```python
from build123d import *

# Parameters (mm, degrees)
SKETCH1_W                       = 152.4
SKETCH1_H                       = 101.6
BOSS_EXTRUDE1_DEPTH             = 46.99
SKETCH2_R                       = 17.145
CUT_EXTRUDE1_DEPTH              = 190.093574983
SKETCH2_2_R                     = 25.4
SKETCH2_2_R_2                   = 17.145
CUT_EXTRUDE3_DEPTH              = 12.446
TAP_DRILL_FOR_1_2_13_TAP1_D     = 10.71626
TAP_DRILL_FOR_1_2_13_TAP1_DEPTH = 19.05
TAP_DRILL_FOR_1_2_13_TAP1_TIP   = 3.219489309
TAP_DRILL_FOR_1_4_20_TAP1_D     = 5.1054
TAP_DRILL_FOR_1_4_20_TAP1_DEPTH = 13.706183098
TAP_DRILL_FOR_1_4_20_TAP1_TIP   = 1.533816902


with BuildPart() as part:
    # Sketch1 → Boss-Extrude1 (new body)
    with BuildSketch(Plane.XY):
        with Locations((76.2, 50.8)):
            Rectangle(SKETCH1_W, SKETCH1_H)
    extrude(amount=BOSS_EXTRUDE1_DEPTH)

    # Sketch2 → Cut-Extrude1 (cut, through all)
    with BuildSketch(Plane(origin=(0, 0, 0), x_dir=(-1, 0, 0), z_dir=(0, 0, -1))):
        with Locations((-76.2, 50.8)):
            Circle(SKETCH2_R)
    extrude(amount=-CUT_EXTRUDE1_DEPTH, mode=Mode.SUBTRACT)

    # Sketch2<2> → Cut-Extrude3 (cut)
    with BuildSketch(Plane(origin=(0, 0, 0), x_dir=(-1, 0, 0), z_dir=(0, 0, -1))):
        with Locations((-76.2, 50.8)):
            Circle(SKETCH2_2_R)
        with Locations((-76.2, 50.8)):
            Circle(SKETCH2_2_R_2, mode=Mode.SUBTRACT)
    cut_extrude3 = extrude(amount=-CUT_EXTRUDE3_DEPTH, mode=Mode.SUBTRACT)

    # Mirror2: Cut-Extrude3 across plane
    add(cut_extrude3.mirror(Plane(origin=(0, 0, 23.495), x_dir=(1, 0, 0), z_dir=(0, 0, -1))), mode=Mode.SUBTRACT)

    # Tap Drill for 1/2-13 Tap1
    with Locations(Plane(origin=(0, 0, 0), x_dir=(-1, 0, 0), z_dir=(0, -1, 0))):
        with Locations((-68.051669078, -23.495), (-29.951669078, -23.495)):
            Hole(TAP_DRILL_FOR_1_2_13_TAP1_D / 2, depth=TAP_DRILL_FOR_1_2_13_TAP1_DEPTH)
            with Locations((0, 0, -(TAP_DRILL_FOR_1_2_13_TAP1_DEPTH + TAP_DRILL_FOR_1_2_13_TAP1_TIP / 2))):  # 118° drill point
                Cone(0, TAP_DRILL_FOR_1_2_13_TAP1_D / 2, TAP_DRILL_FOR_1_2_13_TAP1_TIP, mode=Mode.SUBTRACT)

    # Tap Drill for 1/4-20 Tap1
    with Locations(Plane(origin=(50.8, 101.6, 0), x_dir=(0, 0, -1), z_dir=(0, 1, 0))):
        with Locations((-12.7, -47.625), (-12.7, -3.175)):
            Hole(TAP_DRILL_FOR_1_4_20_TAP1_D / 2, depth=TAP_DRILL_FOR_1_4_20_TAP1_DEPTH)
            with Locations((0, 0, -(TAP_DRILL_FOR_1_4_20_TAP1_DEPTH + TAP_DRILL_FOR_1_4_20_TAP1_TIP / 2))):  # 118° drill point
                Cone(0, TAP_DRILL_FOR_1_4_20_TAP1_D / 2, TAP_DRILL_FOR_1_4_20_TAP1_TIP, mode=Mode.SUBTRACT)


solid = part.part
```
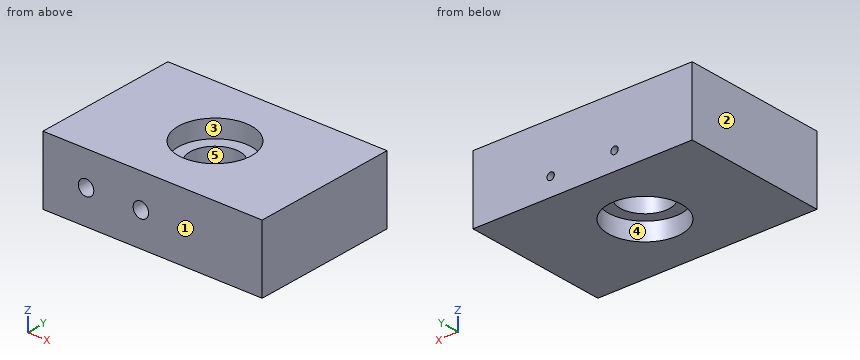
Source: CAD feature listing. Evaluate the final solid. Frame: model axes, mm. Face numbers are marked on the shaded views. A direction names the side the tool comes from. Give positions to 0.01 mm unless a question says otherwise; leave off trailing zeros. Loops run counter-clockwise (first coordinate to the right, second up) from the corner with the lowest first, then second, coordinate; pieces in that order, holes last. Notation, with made-up numbers: (2.25, -13.75) -> (13.25, -13.75) arc R26 cw to (13.25, 21.25) -> close; hole circle Ø3 at (32.5, -1.75). An arc over 180 degrees is marked (long way). Put each result on its own line as item: value. Start each with the question number.
1) Cut plane D-D (y = 6). Return loops of the section in (x, z) (3 decimals).
2) Cut plane A-A (x = 76.2). Return loops of the section in (y, z) (3 decimals).
3) Reachability of the marked faces 4 and 5 from +Z, -Z, +X, -X, +Y, -Y: full face, straight path, thin tool, end or side. Return the list, or none.
4) Cut plane B-B (y = 50.8). Return loops of the section in (x, z) (3 decimals).
5) Contact query for flat-ended pins moving along their axis: P1, Ø6.5, axis at x = 68.05, z = 23.5, coming from the -Y side; P2, Ø5, axis at x = 75, y = 67, coming from the -Z side; P3, Ø4.5, axis at x = 53.975, z = 12.7, coming from the +Y side. Output: stop coordinate, or through.
6) Cut plane C-C (y = 71). Return loops of the section in (x, z).
7) Material intervals for probe 1 along X at (y, z) = (98.75, 12.7); probe 2 along X at (y, z) = (6.5, 23); probe 3 along X at (y, z) = (50, 41), sorted ascending.
8) Draft query along X for the marked faces 1, 2 and 3. Return one class per face: released by +X, released by -X, zero draft, split by the parting line, or undercut.
Results are:
1. outline: (0, 0) -> (152.4, 0) -> (152.4, 46.99) -> (0, 46.99) -> close; hole circle Ø10.716 at (29.952, 23.495); hole circle Ø10.716 at (68.052, 23.495)
2. outline: (0, 0) -> (25.4, 0) -> (25.4, 12.446) -> (33.655, 12.446) -> (33.655, 34.544) -> (25.4, 34.544) -> (25.4, 46.99) -> (0, 46.99) -> close; (67.945, 12.446) -> (76.2, 12.446) -> (76.2, 0) -> (101.6, 0) -> (101.6, 46.99) -> (76.2, 46.99) -> (76.2, 34.544) -> (67.945, 34.544) -> close
3. face 4: -Z
3. face 5: +Z, -Z
4. outline: (0, 0) -> (50.8, 0) -> (50.8, 12.446) -> (59.055, 12.446) -> (59.055, 34.544) -> (50.8, 34.544) -> (50.8, 46.99) -> (0, 46.99) -> close; (93.345, 12.446) -> (101.6, 12.446) -> (101.6, 0) -> (152.4, 0) -> (152.4, 46.99) -> (101.6, 46.99) -> (101.6, 34.544) -> (93.345, 34.544) -> close
5. P1: stops at y = 20.31
5. P2: stops at z = 12.45
5. P3: stops at y = 87.71
6. outline: (0, 0) -> (60.8, 0) -> (60.8, 12.45) -> (91.6, 12.45) -> (91.6, 0) -> (152.4, 0) -> (152.4, 46.99) -> (91.6, 46.99) -> (91.6, 34.54) -> (60.8, 34.54) -> (60.8, 46.99) -> (0, 46.99) -> close
7. probe 1: x = 0 to 51.42, 56.53 to 95.87, 100.98 to 152.4
7. probe 2: x = 0 to 24.62, 35.29 to 62.72, 73.39 to 152.4
7. probe 3: x = 0 to 50.81, 101.59 to 152.4
8. face 1: zero draft
8. face 2: released by -X
8. face 3: undercut
